Autodesk Inventor part; units mm, degrees
ref_plane "YZ Plane" through (0, 0, 0) normal (1, 0, 0) x (0, 1, 0)
ref_plane "XZ Plane" through (0, 0, 0) normal (0, 1, 0) x (-1, 0, 0)
ref_plane "XY Plane" through (0, 0, 0) normal (0, 0, 1) x (1, 0, 0)
sketch "Sketch1" plane through (0, 0, 0) normal (0, 1, 0) x (-1, 0, 0)
  line L0 (-70, 135) -> (-70, -135)
  line L1 (-70, -135) -> (70, -135)
  line L2 (70, -135) -> (70, 135)
  line L3 (70, 135) -> (-70, 135)
  line L4 (-70, 135) -> (70, -135) construction
  line L5 (-70, -135) -> (70, 135) construction
  line L6 (70, 85) -> (20, 135)
  line L7 (-20, 135) -> (-70, 85)
  point P0 (0, 0)
  dimension "d0" = 140
  dimension "d1" = 270
  dimension "d2" = 40
  dimension "d3" = 50
  dimension "d4" = 220
extrude "Extrusion1" add sketch "Sketch1" along normal blind 4.05 and the other way blind 4.05 contours L7 L3 L6 L2 L1 L0
sketch "Sketch2" plane through (0, 0, 0) normal (0, 1, 0) x (-1, 0, 0)
  line L0 (70, -135) -> (70, 85)
  line L1 (70, 85) -> (20, 135)
  line L2 (20, 135) -> (-20, 135)
  line L3 (-20, 135) -> (-70, 85)
  line L4 (-70, 85) -> (-70, -135)
  line L5 (-70, -135) -> (70, -135)
  line L6 (70, 83) -> (30, 83)
  line L7 (30, 83) -> (30, 43)
  line L8 (30, 43) -> (70, 43)
  line L9 (70, 43) -> (70, 83)
  line L10 (70, 85) -> (70, -135)
  line L11 (70, -133) -> (30, -133)
  line L12 (30, -133) -> (30, -93)
  line L13 (30, -93) -> (70, -93)
  line L14 (70, -93) -> (70, -133)
  line L15 (-30, 43) -> (-30, 83)
  line L16 (-70, 43) -> (-30, 43)
  line L17 (-30, 83) -> (-70, 83)
  line L18 (-70, 83) -> (-70, 43)
  line L19 (-30, -93) -> (-30, -133)
  line L20 (-70, -93) -> (-30, -93)
  line L21 (-30, -133) -> (-70, -133)
  line L22 (-70, -133) -> (-70, -93)
  point P0 (0, 0)
  point P1 (50, 83)
  point P2 (50, -133)
  point P3 (-50, 83)
  point P4 (-50, -133)
  dimension "d11" = 40
  dimension "d12" = 40
  dimension "d13" = 2
  dimension "d14" = 2
  dimension "d15" = 40
  dimension "d16" = 40
  dimension "d19" = 100
extrude "Extrusion2" cut sketch "Sketch2" along normal blind 0.75 and the other way blind 0.75 contours L11 L12 L13 L0 | L4 L20 L19 L21 | L8 L7 L6 L0 | L4 L17 L15 L16
sketch "Sketch3" plane through (0, 0, 0) normal (0, 1, 0) x (-1, 0, 0)
  line L0 (70, -135) -> (70, 85)
  line L1 (70, 85) -> (20, 135)
  line L2 (20, 135) -> (-20, 135)
  line L3 (-20, 135) -> (-70, 85)
  line L4 (-70, 85) -> (-70, -135)
  line L5 (-70, -135) -> (70, -135)
  point P0 (0, 0)
extrude "Extrusion3" cut sketch "Sketch3" along normal up to surface (4.05 mm away)
sketch "Sketch5" plane through (0, -4.05, 0) normal (0, -1, 0) x (1, 0, 0)
  line L0 (62, 78) -> (38, 78)
  line L1 (38, 78) -> (38, 48)
  line L2 (38, 48) -> (62, 48)
  line L3 (62, 48) -> (62, 78)
  line L4 (30, -93) -> (70, -93)
  line L5 (30, -133) -> (30, -93)
  line L6 (70, -133) -> (30, -133)
  line L7 (70, -135) -> (70, -133)
  line L8 (-70, -135) -> (70, -135)
  line L9 (-70, -133) -> (-70, -135)
  line L10 (-30, -133) -> (-70, -133)
  line L11 (-30, -93) -> (-30, -133)
  line L12 (-70, -93) -> (-30, -93)
  line L13 (-70, 43) -> (-70, -93)
  line L14 (-30, 43) -> (-70, 43)
  line L15 (-30, 83) -> (-30, 43)
  line L16 (-70, 83) -> (-30, 83)
  line L17 (-70, 85) -> (-70, 83)
  line L18 (-20, 135) -> (-70, 85)
  line L19 (20, 135) -> (-20, 135)
  line L20 (70, 85) -> (20, 135)
  line L21 (70, 83) -> (70, 85)
  line L22 (30, 83) -> (70, 83)
  line L23 (30, 43) -> (30, 83)
  line L24 (70, 43) -> (30, 43)
  line L25 (70, -93) -> (70, 43)
  circle A0 centre (62, 78) radius 1.5
  point P0 (0, 0)
  dimension "d31" = 24
  dimension "d32" = 30
  dimension "d33" = 8
  dimension "d34" = 5
  dimension "d35" = 3
extrude "Extrusion4" cut sketch "Sketch5" against normal up to surface (3.3 mm away) contours L3 A0 L0 | L0 A0 L3
pattern_linear "Rectangular Pattern1" count 2 spacing 30 along (0, 0, -1) count 2 spacing 24 along (-1, 0, 0) of "Extrusion4"
pattern_linear "Rectangular Pattern2" count 2 spacing 176 along (0, 0, -1) count 2 spacing 100 along (-1, 0, 0) of "Extrusion4", "Rectangular Pattern1"
sketch "Sketch6" plane through (0, -4.05, 0) normal (0, -1, 0) x (1, 0, 0)
  line L0 (18.5, -84) -> (-18.5, -84)
  line L1 (-18.5, -84) -> (-18.5, 8)
  line L2 (-18.5, 8) -> (18.5, 8)
  line L3 (18.5, 8) -> (18.5, -84)
  line L4 (70, -93) -> (70, 43)
  line L5 (70, 13) -> (-70, 13)
  line L6 (-70, 85) -> (-70, -135)
  line L7 (-70, -135) -> (70, -135)
  circle A0 centre (18.5, 8) radius 1.5
  point P0 (0, 0)
  point P1 (0, 8)
  dimension "d50" = 148
  dimension "d51" = 5
  dimension "d52" = 92
  dimension "d53" = 37
  dimension "d54" = 3
extrude "Extrusion5" cut sketch "Sketch6" against normal up to next contours A0 L2 L3 | L3 L2 A0
pattern_linear "Rectangular Pattern3" count 5 spacing 23 along (0, 0, -1) count 2 spacing 37 along (-1, 0, 0) of "Extrusion5"
sketch "Sketch7" plane through (0, -4.05, 0) normal (0, -1, 0) x (1, 0, 0)
  line L0 (70, -135) -> (70, 85)
  line L1 (-70, 85) -> (-70, -135)
  line L2 (-70, -135) -> (70, -135)
  circle A0 centre (62.5, -80) radius 1.5
  circle A1 centre (-62.5, -80) radius 1.5
  point P0 (0, 0)
  dimension "d63" = 7.5
  dimension "d64" = 7.5
  dimension "d65" = 55
  dimension "d66" = 55
  dimension "d67" = 3
  dimension "d68" = 3
extrude "Extrusion6" cut sketch "Sketch7" against normal up to next
pattern_linear "Rectangular Pattern4" count 8 spacing 15 along (0, 0, 1) of "Extrusion6"
properties part number "low_base"
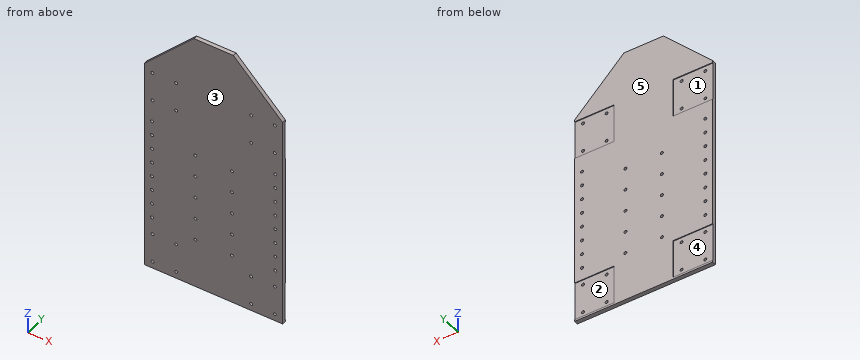
Here's how the part is built. I have some questions about the finished solid (model axes, mm). Face numbers are marked on the shaded views. A direction names the side the tool comes from. Give positions to 0.01 mm unless a question says otherwise; leave off trailing zeros. Write each loop counter-clockwise with the first axis right and the second up, starting at its lowest first coordinate (ties: lowest second). Pieces come first, ordered by that corner, then holes. Notation, with made-up numbers: (84.5, 39) -> (128.5, 39) arc R27 ccw to (128.5, 77) -> close; hole circle Ø5 at (-37, -32). An arc over 180 degrees is marked (long way). Use one line per item in the form item = value. Start each with the question number.
1. Thinking about a two-plate mould opening in Z: for the marked faces 4 and 5, which applies, +Z half, -Z half, draft (parallel to the pull), parting line (faces both ways), or undercut?
2. Imagine slicing it at B-B on z = -116. List the corners of the cut face in (x, y) for me, plus the area to 3 significant figures.
3. Imagine slicing it at C-C on y = -3. State how many separate pieces and enclosed holes the cut face has, plus the area to 3 significant figures.
4. On a 3-axis mill with a long thin cutter (end or side, diameter ignored), from which of +Z, -Z, +X, -X, +Y, -Y can I reach the whole of each face in a straight line? I mean the marked faces 1, 2 and 3. Say none if no direction works.
5. If I drill on L1, parallel to Z at x = -18.5, y = -1.85; L2, parallel to X at y = -1.25, z = -84; L3, parallel to X at y = -2.9, z = 78, over which ranges is the centre line in solid material (lowest first)?
6. Will these pins go through, and if not, where does the flat tip stop? pin 1 Ø5 at (x, z) = (38, 78) entering from +Y; pin 2 Ø1 at (x, y) = (54, -2.5) entering from +Z; pin 3 Ø0.8 at (x, y) = (-43, -0.5) entering from +Z.
7. Imagine slicing it at A-A on x = -58. List the corners of the cut face in (y, z) for me.
Entries:
q1.face_4 = undercut
q1.face_5 = draft
q2.outline = (-70, -4.05) -> (70, -4.05) -> (70, -0.75) -> (30, -0.75) -> (30, 0) -> (-30, 0) -> (-30, -0.75) -> (-70, -0.75) -> close
q2.area = 507 mm²
q3.separate_pieces = 1
q3.enclosed_holes = 42
q3.area = 35,000 mm²
q4.face_1 = -X, +Y
q4.face_2 = +X, +Y
q4.face_3 = +Z, -Z, +X, -X, -Y
q5.L1 = -135 to -85.5, -82.5 to -62.5, -59.5 to -39.5, -36.5 to -16.5, -13.5 to 6.5, 9.5 to 135
q5.L2 = -70 to -20, -17 to 17, 20 to 70
q5.L3 = -70 to -63.5, -60.5 to -39.5, -36.5 to 36.5, 39.5 to 60.5, 63.5 to 70
q6.pin_1 = -0.75
q6.pin_2 = 101.5
q6.pin_3 = 112.4
q7.outline = (-4.05, -135) -> (0, -135) -> (0, -133) -> (-0.75, -133) -> (-0.75, -93) -> (0, -93) -> (0, 43) -> (-0.75, 43) -> (-0.75, 83) -> (0, 83) -> (0, 97) -> (-4.05, 97) -> close
